The model under review builds one solid part; all positions refer to its coordinate system, in mm. A direction names the side the tool comes from. Coordinates: 2 decimals unless noted, no trailing zeros. Loops run counter-clockwise (first coordinate to the right, second up) from the corner with the lowest first, then second, coordinate; pieces in that order, holes last. Notation, with made-up numbers: (21.5, -27) - (72.5, -27) arc R14 ccw to (72.5, -20) - close; hole circle Ø10 at (-12.75, 55). An arc over 180 degrees is marked (long way). Use a Markdown table: item, result. Add a question column.
1) To check wall thickness, follow L1, parallel to X at y = 31.75, z = 0.65; L2, parallel to X at y = 16.5, z = 4.2; L3, parallel to Z at x = -8, y = 20.75. State the ranges of each line that lie inside material, in increasing order. Write a range as [from, to].
2) Add section D-D, the plane x = 43. Give the boundary of the cut face in (y, z), and give its area (3 significant figures).
3) Add section B-B, the plane x = 14. Give the boundary of the cut face in (y, z).
4) The part is to be moulded in two halves that separate along Y. For faces 6 (the cylindrical face through (-10.72, 21.98, 1.48)), 7 (the flat face through (-30.678, 32, 1)), 8 (the flat face through (13, 31.272, 1)), say which applies: pulls with the +Y half, pulls with the -Y half, needs draft (parallel to the pull), parting line crosses it, or undercut.
5) Add section C-C, the plane y = 28.5. Give the boundary of the cut face in (x, z), and give its area (3 significant figures).
6) Add section A-A, the plane z = 0.95. Give the boundary of the cut face in (x, y), and give its area (3 significant figures).
7) For faces 1 (the flat face through (-40.678, 9, 1)), 2 (the flat face through (-38.678, 28, 1)), 3 (the flat face through (61, 33.272, 1)), 4 (the flat face through (6.822, 32, 1)), 5 (the cylindrical face through (15.753, 15.622, 3.986)), list the 3-axis set-ups (+Z, -Z, +X, -X, +Y, -Y) from which the entire face can be reached by the end or side of a thin tool; tool diameter is ignored.
8) Clearance check with flat-ended pins moving along their axes: pin 1 (1.5 mm diameter, centred on y = 27.5, z = 2, fed in from -X); pin 2 (2.5 mm diameter, centred on x = -23, z = 1.5, fed in from +Y); pin 3 (1.8 mm diameter, centred on x = 31.82, y = 15.17, fed in from +Z). State where each tip first meets the part, or that it passes through.
```python
from build123d import *

# Parameters (mm, degrees)
ESBO_O1_R                = 3
ESBO_O1_R_2              = 1.5
RESSALTO_EXTRUS_O1_DEPTH = 3
ESBO_O1_19_R             = 3.5
ESBO_O1_19_R_2           = 1.5
RESSALTO_EXTRUS_O2_DEPTH = 5
ESBO_O1_20_R             = 1.5
RESSALTO_EXTRUS_O3_DEPTH = 3


with BuildPart() as part:
    # Esboço1 → Ressalto-extrusão1 (new body)
    with BuildSketch(Plane.XY):
        Polygon((-30.67768595, 33.271694215), (-40.67768595, 33.271694215), (-40.67768595, 31.271694215), (-38.67768595, 31.271694215), (-38.67768595, 25.271694215), (-40.67768595, 25.271694215), (-40.67768595, 16.271694215), (-38.67768595, 16.271694215), (-38.67768595, 10.271694215), (-40.67768595, 10.271694215), (-40.67768595, 8.271694215), (66.32231405, 8.271694215), (66.32231405, 33.271694215), (56.32231405, 33.271694215), (56.32231405, 31.271694215), (44.32231405, 31.271694215), (44.32231405, 33.271694215), (18.82231405, 33.271694215), (18.82231405, 31.271694215), (6.82231405, 31.271694215), (6.82231405, 33.271694215), (-18.67768595, 33.271694215), (-18.67768595, 31.271694215), (-30.67768595, 31.271694215), align=None)
        with Locations((-12.336122998, 19.452784517)):
            Circle(ESBO_O1_R, mode=Mode.SUBTRACT)
        with Locations((14.32231405, 15.171694215)):
            Circle(ESBO_O1_R_2, mode=Mode.SUBTRACT)
        with Locations((31.82231405, 15.171694215)):
            Circle(ESBO_O1_R_2, mode=Mode.SUBTRACT)
    extrude(amount=RESSALTO_EXTRUS_O1_DEPTH)

    # Esboço1<19> → Ressalto-extrusão2 (add)
    with BuildSketch(Plane.XY):
        with Locations((14.32231405, 15.171694215)):
            Circle(ESBO_O1_19_R)
        with Locations((14.32231405, 15.171694215)):
            Circle(ESBO_O1_19_R_2, mode=Mode.SUBTRACT)
        with Locations((31.82231405, 15.171694215)):
            Circle(ESBO_O1_19_R)
        with Locations((31.82231405, 15.171694215)):
            Circle(ESBO_O1_19_R_2, mode=Mode.SUBTRACT)
    extrude(amount=RESSALTO_EXTRUS_O2_DEPTH)

    # Esboço1<20> → Ressalto-extrusão3 (add)
    with BuildSketch(Plane.XY):
        with Locations((14.32231405, 15.171694215)):
            Circle(ESBO_O1_20_R)
        with Locations((31.82231405, 15.171694215)):
            Circle(ESBO_O1_20_R)
    extrude(amount=RESSALTO_EXTRUS_O3_DEPTH)


solid = part.part
```
From the geometry:
| question | item | result |
|---|---|---|
| 1 | L1 | x = [-40.68, -30.68], [-18.68, 6.82], [18.82, 44.32], [56.32, 66.32] |
| 1 | L2 | x = [11.08, 13.63], [15.02, 17.56], [28.58, 31.13], [32.52, 35.06] |
| 1 | L3 | z = [0, 3] |
| 2 | outline | (8.27, 0) - (33.27, 0) - (33.27, 3) - (8.27, 3) - close |
| 2 | area | 75.0 mm^2 |
| 3 | outline | (8.27, 0) - (31.27, 0) - (31.27, 3) - (18.66, 3) - (18.66, 5) - (16.64, 5) - (16.64, 3) - (13.71, 3) - (13.71, 5) - (11.69, 5) - (11.69, 3) - (8.27, 3) - close |
| 4 | face 6 | undercut |
| 4 | face 7 | needs draft |
| 4 | face 8 | pulls with the +Y half |
| 5 | outline | (-38.68, 0) - (66.32, 0) - (66.32, 3) - (-38.68, 3) - close |
| 5 | area | 315 mm^2 |
| 6 | outline | (-40.68, 8.27) - (66.32, 8.27) - (66.32, 33.27) - (56.32, 33.27) - (56.32, 31.27) - (44.32, 31.27) - (44.32, 33.27) - (18.82, 33.27) - (18.82, 31.27) - (6.82, 31.27) - (6.82, 33.27) - (-18.68, 33.27) - (-18.68, 31.27) - (-30.68, 31.27) - (-30.68, 33.27) - (-40.68, 33.27) - (-40.68, 31.27) - (-38.68, 31.27) - (-38.68, 25.27) - (-40.68, 25.27) - (-40.68, 16.27) - (-38.68, 16.27) - (-38.68, 10.27) - (-40.68, 10.27) - close; hole circle Ø6 at (-12.34, 19.45) |
| 6 | area | 2,550 mm^2 |
| 7 | face 1 | +Z, -Z, -X, +Y, -Y |
| 7 | face 2 | +Z, -Z, -X |
| 7 | face 3 | +Z, -Z, +X, -X, +Y |
| 7 | face 4 | +Z, -Z, +Y |
| 7 | face 5 | +Z |
| 8 | pin 1 | stops at x = -38.68 |
| 8 | pin 2 | stops at y = 31.27 |
| 8 | pin 3 | stops at z = 3 |
